from build123d import *

# Parameters (mm, degrees)
F0_R     = 3.175
F0_R_2   = 1.5875
F1_DEPTH = 3.048


with BuildPart() as f1:
    # F0 (on Front) → F1 (new body)
    with BuildSketch(Plane.XZ):
        with BuildLine():
            ThreePointArc((44.44426, -7.937498), (50.06063, -5.614689), (52.3875, 0))
            ThreePointArc((52.3875, 0), (50.06063, 5.614689), (44.44426, 7.937498))
            ThreePointArc((44.44426, 7.937498), (36.5125, 0), (44.44426, -7.937498))
        make_face()
        with Locations((44.45, 0)):
            Circle(F0_R, mode=Mode.SUBTRACT)
        with BuildLine():
            ThreePointArc((44.44426, -7.937498), (36.5125, 0), (44.44426, 7.937498))
            Line((44.44426, 7.937498), (17.949427, 7.918338))
            ThreePointArc((17.949427, 7.918338), (11.978937, 10.612345), (10.057351, 16.874287))
            Line((10.057351, 16.874287), (15.747457, 61.491711))
            ThreePointArc((15.747457, 61.491711), (0, 47.625), (-15.747457, 61.491711))
            Line((-15.747457, 61.491711), (-7.905356, 0))
            ThreePointArc((-7.905356, 0), (0, 7.905356), (7.905356, 0))
            ThreePointArc((7.905356, 0), (5.589931, -5.589931), (0, -7.905356))
            Line((0, -7.905356), (44.44426, -7.937498))
        make_face()
        with BuildLine():
            ThreePointArc((-7.905356, 0), (-5.589931, -5.589931), (0, -7.905356))
            ThreePointArc((0, -7.905356), (5.589931, -5.589931), (7.905356, 0))
            ThreePointArc((7.905356, 0), (0, 7.905356), (-7.905356, 0))
        make_face()
        Circle(F0_R, mode=Mode.SUBTRACT)
        with BuildLine():
            ThreePointArc((-15.747457, 61.491711), (0, 47.625), (15.747457, 61.491711))
            ThreePointArc((15.747457, 61.491711), (15.843082, 62.493832), (15.875, 63.5))
            ThreePointArc((15.875, 63.5), (15.843082, 64.506168), (15.747457, 65.508289))
            ThreePointArc((15.747457, 65.508289), (0, 79.375), (-15.747457, 65.508289))
            ThreePointArc((-15.747457, 65.508289), (-15.875, 63.5), (-15.747457, 61.491711))
        make_face()
        with Locations((0, 63.5)):
            Circle(F0_R, mode=Mode.SUBTRACT)
        with BuildLine():
            Line((-9.525, 114.3), (-15.747457, 65.508289))
            ThreePointArc((-15.747457, 65.508289), (0, 79.375), (15.747457, 65.508289))
            Line((15.747457, 65.508289), (9.525, 114.3))
            ThreePointArc((9.525, 114.3), (0, 104.775), (-9.525, 114.3))
        make_face()
        with Locations((-6.298599, 100.0252)):
            Circle(F0_R_2, mode=Mode.SUBTRACT)
        with BuildLine():
            ThreePointArc((9.525, 114.3), (0, 123.825), (-9.525, 114.3))
            ThreePointArc((-9.525, 114.3), (0, 104.775), (9.525, 114.3))
        make_face()
        with Locations((0, 114.3)):
            Circle(F0_R, mode=Mode.SUBTRACT)
    extrude(amount=F1_DEPTH)


solid = f1.part
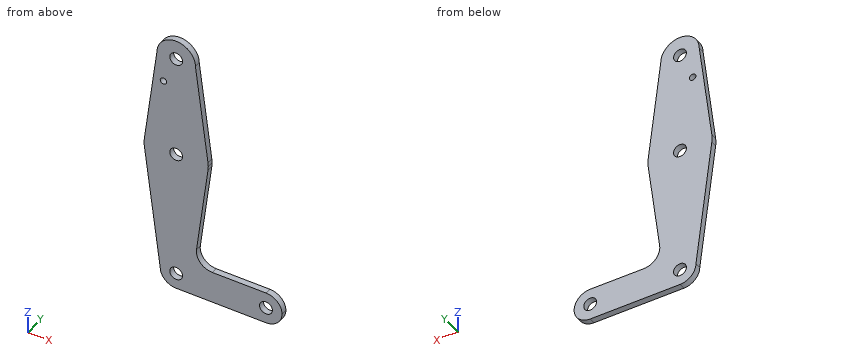
Verification items for the finished model (mm, model axes). Give positions to 0.01 mm unless a question says otherwise; leave off trailing zeros. Write each loop counter-clockwise with the first axis right and the second up, starting at its lowest first coordinate (ties: lowest second). Pieces come first, ordered by that corner, then holes. Notation, with made-up numbers: (-35, 30.25) - (-8, 30.25) arc R20 ccw to (-8, 43.25) - close; hole circle Ø9 at (-6.5, -31.5). An arc over 180 degrees is marked (long way). Answer as CSV lines item,"result". Start each with the question number.
1. Sectioned sample at A-A (x = 42.5). Record the boundary of the cut face in (y, z).
2. Sectioned sample at C-C (y = -2.25). Count the separate pieces of the cut face and the enclosed holes in it, then the cut area to 3 significant figures.
3. Sectioned sample at B-B (x = -1.5). Record the boundary of the cut face in (y, z).
4. Thickness scan on line 1 (Z direction, x = 44.45, y = -0.7) (1 decimal); line 2 (Z direction, x = 23.5, y = -2.25); line 3 (X direction, y = -1.2, z = -1). Record the ranges inside material, lowest first.
5. Depth check by flat-ended pin: pin 1 (1 mm diameter, centred on x = 2.5, y = -2, fed in from +Z). Enter the tip coordinate at first touch or a pass-through.
6. Sectioned sample at D-D (z = 97). Record the boundary of the cut face in (x, y), then the cut area to 3 significant figures.
Derived:
1,outline,"(-3.05, -7.94) - (0, -7.94) - (0, -2.51) - (-3.05, -2.51) - close; (-3.05, 2.51) - (0, 2.51) - (0, 7.94) - (-3.05, 7.94) - close"
2,separate pieces,"1"
2,enclosed holes,"5"
2,area,"3,630 mm²"
3,outline,"(-3.05, -7.76) - (0, -7.76) - (0, -2.8) - (-3.05, -2.8) - close; (-3.05, 2.8) - (0, 2.8) - (0, 60.7) - (-3.05, 60.7) - close; (-3.05, 66.3) - (0, 66.3) - (0, 111.5) - (-3.05, 111.5) - close; (-3.05, 117.1) - (0, 117.1) - (0, 123.71) - (-3.05, 123.71) - close"
4,line 1,"-7.9 to -3.2, 3.2 to 7.9"
4,line 2,"-7.92 to 7.92"
4,line 3,"-7.84 to -3.01, 3.01 to 41.44, 47.46 to 52.32"
5,pin 1,"z = 123.61"
6,outline,"(-11.73, -3.05) - (11.73, -3.05) - (11.73, 0) - (-11.73, 0) - close"
6,area,"71.5 mm²"
